```python
from build123d import *

# Parameters (mm, degrees)
SKETCH2_R                  = 3.175
BOSS_EXTRUDE1_DEPTH        = 4.7625
BOSS_EXTRUDE2_START        = 11.1125
BOSS_EXTRUDE2_DEPTH        = 11.1125
SKETCH12_W                 = 6.477
SKETCH12_H                 = 13.919150617
SKETCH12_H_2               = 7.9375
CUT_EXTRUDE1_DEPTH         = 24.13
SKETCH12_3_W               = 6.477
SKETCH12_3_H               = 4.7625
CUT_EXTRUDE2_DEPTH         = 19.05
TAP_DRILL_FOR_10_32_TAP1_D = 4.0386
F_10_CLEARANCE_HOLE2_D     = 4.9784


with BuildPart() as part:
    # Sketch2 → Boss-Extrude1 (new body)
    with BuildSketch(Plane.XY):
        with BuildLine():
            Line((-67.986186343, -228.533359856), (-69.686856366, -224.252380141))
            Line((-69.686856366, -224.252380141), (-61.0470258, -221.260552334))
            Line((-61.0470258, -221.260552334), (-48.895, -221.260552334))
            Line((-48.895, -221.260552334), (-48.895, -203.133359856))
            ThreePointArc((-48.895, -203.133359856), (-45.175256121, -194.153103735), (-36.195, -190.433359856))
            Line((-36.195, -190.433359856), (25.4, -190.433359856))
            Line((25.4, -190.433359856), (25.4, -228.533359856))
            Line((25.4, -228.533359856), (-67.986186343, -228.533359856))
        make_face()
        with Locations(Location((-36.195, -203.133359856, 0), (0, 0, 180))):
            Circle(SKETCH2_R, mode=Mode.SUBTRACT)
    extrude(amount=BOSS_EXTRUDE1_DEPTH)

    # Sketch11 → Boss-Extrude2 (add)
    with BuildSketch(Plane(origin=(0, 0, 0), x_dir=(-1, 0, 0), z_dir=(0, 0, -1)).offset(BOSS_EXTRUDE2_START)):
        with BuildLine():
            Line((25.4, -190.433359856), (25.4, -228.533359856))
            Line((25.4, -228.533359856), (67.986186343, -228.533359856))
            Line((67.986186343, -228.533359856), (69.686856366, -224.252380141))
            Line((69.686856366, -224.252380141), (61.0470258, -221.260552334))
            Line((61.0470258, -221.260552334), (48.895, -221.260552334))
            Line((48.895, -221.260552334), (48.895, -203.133359856))
            ThreePointArc((48.895, -203.133359856), (45.175256121, -194.153103735), (36.195, -190.433359856))
            Line((36.195, -190.433359856), (25.4, -190.433359856))
        make_face()
    extrude(amount=-BOSS_EXTRUDE2_DEPTH)

    # Sketch12 → Cut-Extrude1 (cut)
    with BuildSketch(Plane.ZY.offset(48.895)):
        with Locations((-3.2385, -210.092935165)):
            Rectangle(SKETCH12_W, SKETCH12_H)
        with Locations((-3.2385, -199.164609856)):
            Rectangle(SKETCH12_W, SKETCH12_H_2)
    extrude(amount=-CUT_EXTRUDE1_DEPTH, mode=Mode.SUBTRACT)

    # Sketch12_3 → Cut-Extrude2 (cut)
    with BuildSketch(Plane.ZY.offset(48.895)):
        with Locations((-3.2385, -192.814609856)):
            Rectangle(SKETCH12_3_W, SKETCH12_3_H)
    extrude(amount=-CUT_EXTRUDE2_DEPTH, mode=Mode.SUBTRACT)

    # Tap Drill for _10-32 Tap1 (through all)
    with Locations(Plane.XY.offset(-6.477)):
        with Locations((-36.195, -203.133359856)):
            Hole(TAP_DRILL_FOR_10_32_TAP1_D / 2)

    # 10 Clearance Hole2 (through all)
    with Locations(Plane.XY.offset(4.7625)):
        with Locations((-10.8204, -196.783359856), (-10.8204, -222.183359856), (10.8204, -222.183359856), (10.8204, -196.783359856)):
            Hole(F_10_CLEARANCE_HOLE2_D / 2)


solid = part.part
```
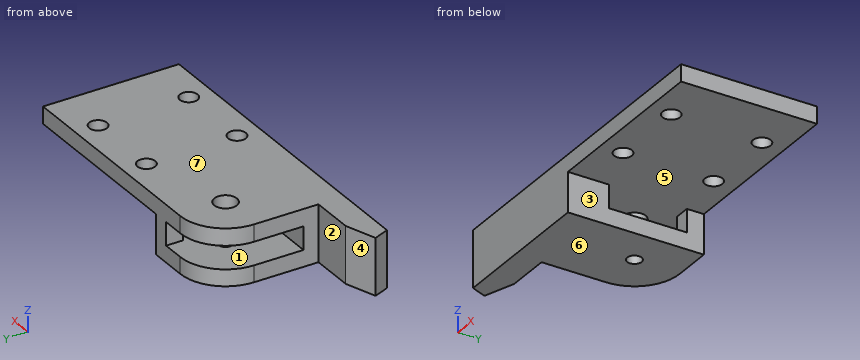
Check sheet for the modelled part. Datum: model origin and axes. Units: mm. Face numbers are marked on the shaded views. A direction names the side the tool comes from. Round coordinates to 2 decimals unless told otherwise and drop trailing zeros. Order: outer loops, then holes, each group sorted by start corner. A loop starts at its lowest first (then second) coordinate and runs counter-clockwise, first axis right, second up. Notation, with made-up numbers: (88.25, 85) - (115.25, 85) arc R14 cw to (115.25, 94) - close; hole circle Ø2 at (37.5, 66). An arc over 180 degrees is marked (long way). Answer as CSV lines item,"result". Start each with the question number.
1) Section check A-A (z = -7.5). Record the cut outline in (x, y) (3 decimals), then the cut area to 3 significant figures.
2) Section check B-B (z = -2). Record the cut outline in (x, y) (3 decimals), then the cut area to 3 significant figures.
3) Section check D-D (y = -212). Record the cut outline in (x, z) (1 decimal).
4) Draft check along Z on the marked faces 4, 5, 6 and 7. Enter one of: +Z half, -Z half, draft (parallel to the pull), parting line (faces both ways), or undercut.
5) Scan lines: probe 1 along Z at (x, y) = (-34.5, -193.5); probe 2 along X at (y, z) = (-203.5, 3.25) (3 decimals); probe 3 along Y at (x, z) = (-46.5, -2). Record each from-to range of solid material in increasing order.
6) Depth check by flat-ended pin: pin 1 (5.5 mm diameter, centred on x = -10.82, y = -196.78, fed in from -Z); pin 2 (3 mm diameter, centred on x = -32, z = -4, fed in from +Y); pin 3 (4 mm diameter, centred on y = -193.5, z = -4, fed in from -X) (3 decimals). Enter the tip coordinate at first touch or a pass-through.
7) Section check C-C (x = -27). Record the cut outline in (y, z), then the cut area to 3 significant figures.
8) Tool access check on the marked faces 1, 2 and 3. Record the directions out of +Z, -Z, +X, -X, +Y, -Y that give a thin tool (end or side, any length) a straight path to the whole face; none if there is none.
Determined:
1,outline,"(-69.687, -224.252) - (-67.986, -228.533) - (-25.4, -228.533) - (-25.4, -190.433) - (-36.195, -190.433) arc R12.7 ccw to (-48.895, -203.133) - (-48.895, -221.261) - (-61.047, -221.261) - close; hole circle Ø4.039 at (-36.195, -203.133)"
1,area,"982 mm^2"
2,outline,"(-69.687, -224.252) - (-67.986, -228.533) - (-25.4, -228.533) - (-25.4, -217.053) - (-48.895, -217.053) - (-48.895, -221.261) - (-61.047, -221.261) - close; (-29.845, -195.196) - (-25.4, -195.196) - (-25.4, -190.433) - (-29.845, -190.433) - close"
2,area,"426 mm^2"
3,outline,"(-48.9, -11.1) - (-25.4, -11.1) - (-25.4, -6.5) - (-48.9, -6.5) - close; (-48.9, 0) - (25.4, 0) - (25.4, 4.8) - (-48.9, 4.8) - close"
4,face 4,"draft"
4,face 5,"undercut"
4,face 6,"-Z half"
4,face 7,"+Z half"
5,probe 1,"-11.11 to -6.48, 0 to 4.76"
5,probe 2,"-48.895 to -39.349, -33.041 to 25.4"
5,probe 3,"-228.53 to -217.05"
6,pin 1,"z = 0"
6,pin 2,"y = -217.05"
6,pin 3,"x = -29.845"
7,outline,"(-228.53, -11.11) - (-190.43, -11.11) - (-190.43, 4.76) - (-228.53, 4.76) - close; hole (-217.05, -6.48) - (-195.2, -6.48) - (-195.2, 0) - (-217.05, 0) - close"
7,area,"463 mm^2"
8,face 1,"-X"
8,face 2,"+Z, -Z, -X, +Y"
8,face 3,"-Z, +X, +Y, -Y"
